For this review, use the dimensioned drawing (mm, ordinates from the lowest corner) and the shaded views. A direction names the side the tool comes from. Round coordinates to 2 decimals unless told otherwise and drop trailing zeros. Loops run counter-clockwise (first coordinate to the right, second up) from the corner with the lowest first, then second, coordinate; pieces in that order, holes last. Notation, with made-up numbers: M 86.5,22.25 L 128.5,22.25 A30 ccw 128.5,52.25 Z; hole C 58.5,77.5 d1. An arc over 180 degrees is marked long. Answer as a JSON object with one key per item and string values. Group by question number.
Item 1: Consider section D-D (x = 18). Give the boundary of the cut face in (y, z).
Item 2: Consider section A-A (z = 10). Give the boundary of the cut face in (x, y).
Item 3: Insertion check: P1, Ø2, axis at x = 8, y = 12, coming from the -Z side; P2, Ø1.5, axis at x = 14, z = 15.5, coming from the +Y side. Each pin has a flat end and moves straight along its axis. Give the tip position at first contact, or say it passes through.
Item 4: Consider section C-C (y = 11.74). Give the boundary of the cut face in (x, z), and give its area (3 significant figures).
Item 5: Consider section B-B (x = 4.25). Give the boundary of the cut face in (y, z).
Item 6: To check wall thickness, follow line 1 (X direction, y = 1.9, z = 10); line 2 (Y direction, x = 4.25, z = 29.75); line 3 (Z direction, x = 17, y = 8). State the ranges of each line that lie inside material, in increasing order.
Item 7: Tool access review of the marked faces 1 and 2: name each direction out of +Z, -Z, +X, -X, +Y, -Y from which nothing blocks a thin tool from reaching the whole face with its end or side.
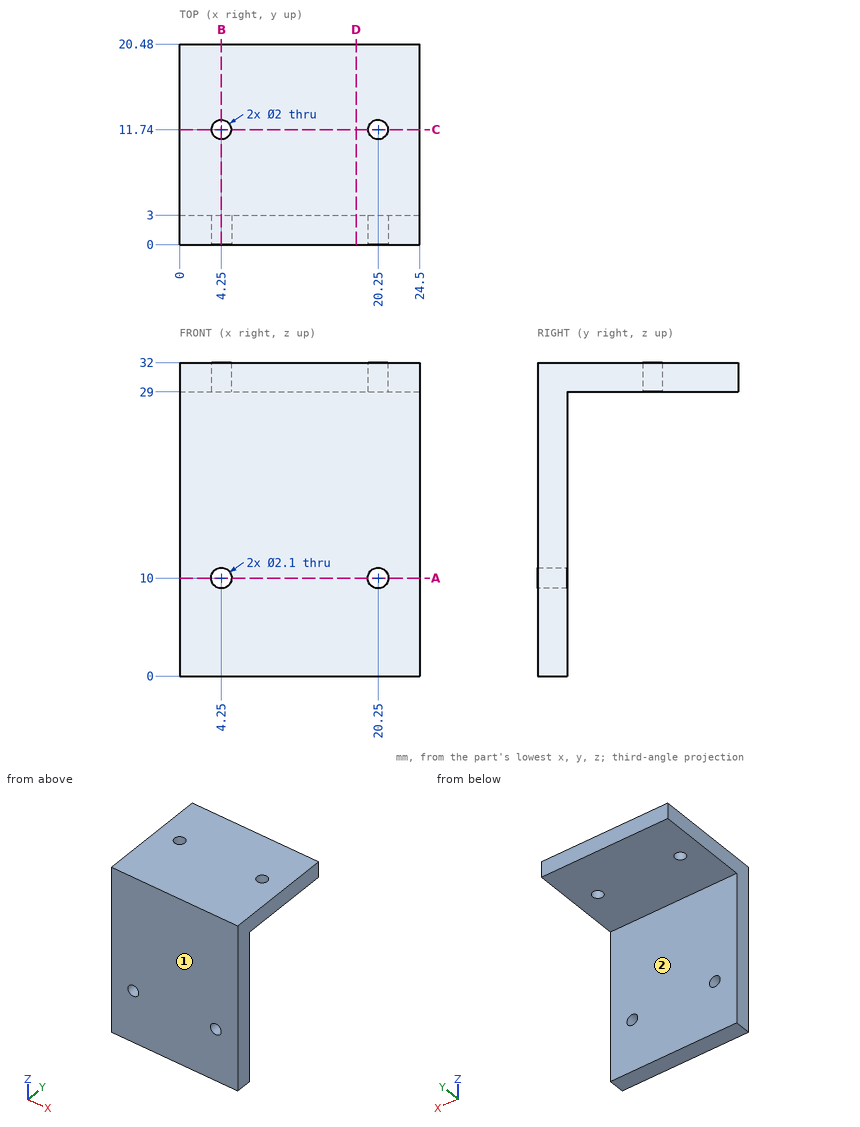
Geometry results:
{
 "1": {"outline": "M 0,0 L 3,0 L 3,29 L 20.48,29 L 20.48,32 L 0,32 Z"},
 "2": {"outline": "M 0,0 L 3.2,0 L 3.2,3 L 0,3 Z; M 5.3,0 L 19.2,0 L 19.2,3 L 5.3,3 Z; M 21.3,0 L 24.5,0 L 24.5,3 L 21.3,3 Z"},
 "3": {"P1": "stops at z = 29", "P2": "stops at y = 3"},
 "4": {"outline": "M 0,29 L 3.25,29 L 3.25,32 L 0,32 Z; M 5.25,29 L 19.25,29 L 19.25,32 L 5.25,32 Z; M 21.25,29 L 24.5,29 L 24.5,32 L 21.25,32 Z", "area": "61.5 mm^2"},
 "5": {"outline": "M 0,0 L 3,0 L 3,8.95 L 0,8.95 Z; M 0,11.05 L 3,11.05 L 3,29 L 10.74,29 L 10.74,32 L 0,32 Z; M 12.74,29 L 20.48,29 L 20.48,32 L 12.74,32 Z"},
 "6": {"line 1": "x = 0 to 3.2, 5.3 to 19.2, 21.3 to 24.5", "line 2": "y = 0 to 10.74, 12.74 to 20.48", "line 3": "z = 29 to 32"},
 "7": {"face 1": "+Z, -Z, +X, -X, -Y", "face 2": "-Z, +X, -X, +Y"}
}
